```python
from build123d import *

# Parameters (mm, degrees)
F0_W     = 83
F0_H     = 60
F1_DEPTH = 25
F2_R     = 5
F3_SIZE  = 10
F5_D     = 4.2
F6_W     = 9.244158864
F6_H     = 29.9456948414
F7_DEPTH = 30
F8_W     = 29.5899156481
F8_H     = 11.4948265254
F9_DEPTH = 15


with BuildPart() as f1:
    # F0 (on Top) → F1 (new body)
    with BuildSketch(Plane.XY):
        with Locations((41.5, 30)):
            Rectangle(F0_W, F0_H)
    extrude(amount=F1_DEPTH)

    # F2
    f2_edges = [f1.edges().sort_by_distance(p)[0] for p in [
        (41.5, 0, 25),
    ]]
    fillet(f2_edges, radius=F2_R)

    # F3
    f3_edges = [f1.edges().sort_by_distance(p)[0] for p in [
        (41.5, 60, 25),
    ]]
    chamfer(f3_edges, length=F3_SIZE)

    # F5 (through all)
    with Locations(Plane.XY.offset(25)):
        with Locations((41.1825105548, 21.0945475847)):
            Hole(F5_D / 2)

    # F6 (on face) → F7 (cut)
    with BuildSketch(Plane.XY.offset(25)):
        with Locations((64.5809471607, 27.1079088561)):
            Rectangle(F6_W, F6_H)
    extrude(amount=-F7_DEPTH, mode=Mode.SUBTRACT)

    # F8 (on face) → F9 (cut)
    with BuildSketch(Plane.XY.offset(25)):
        with Locations((14.7949578241, 18.5050182045)):
            Rectangle(F8_W, F8_H)
    extrude(amount=-F9_DEPTH, mode=Mode.SUBTRACT)


solid = f1.part
```
Geometry check sheet. Reference: the model listing, model coordinates, mm. A direction names the side the tool comes from. Give positions to 0.01 mm unless a question says otherwise; leave off trailing zeros. Order: outer loops, then holes, each group sorted by start corner. A loop starts at its lowest first (then second) coordinate and runs counter-clockwise, first axis right, second up.
1. Section check D-D, the plane x = 25.5. Enter the section's corners in (y, z), and give its area (3 significant figures).
2. Section check B-B, the plane x = 68. Enter the section's corners in (y, z).
3. Section check C-C, the plane z = 18.5. Enter the section's corners in (x, y).
4. Access from +Z, -Z, +X, -X, +Y, -Y to the whole of each face (thin tool, end or side, straight path). Record for faces 4 (the face through (15, 12.758, 18)), 5 (the face through (83, 30, 12)), 6 (the face through (65, 42.081, 13)).
5. Thickness scan on L1, parallel to X at y = 23.5, z = 22.75; L2, parallel to X at y = 31, z = 4.75; L3, parallel to Y at x = 28.5, z = 11.5. Record the ranges inside material, lowest first.
6. Section check A-A, the plane y = 31. Enter the section's corners in (x, z).
7. Gauge pin test, flat ends, axial feed: pin 1 Ø4 at (x, z) = (49, 19.5) entering from +Y; pin 2 Ø3.5 at (x, y) = (15.5, 16) entering from +Z; pin 3 Ø2 at (x, y) = (56, 51.5) entering from +Z. Record the tip position at first contact, or that the pin passes through.
8. Release check for a two-part mould opening along Y. For faces 1 (the face through (42, 1, 23)), 2 (the face through (41, 60, 7)), 3 (the face through (15, 19, 10)) record: pulls with the +Y half, pulls with the -Y half, needs draft (parallel to the pull), parting line crosses it, or undercut.
Values follow:
1. outline: (0, 0) - (60, 0) - (60, 15) - (50, 25) - (24.25, 25) - (24.25, 10) - (12.76, 10) - (12.76, 25) - (5, 25) arc R5 ccw to (0, 20) - close
1. area: 1,270 mm2
2. outline: (0, 0) - (12.14, 0) - (12.14, 25) - (5, 25) arc R5 ccw to (0, 20) - close; (42.08, 0) - (60, 0) - (60, 15) - (50, 25) - (42.08, 25) - close
3. outline: (0, 0) - (83, 0) - (83, 56.5) - (0, 56.5) - (0, 24.25) - (29.59, 24.25) - (29.59, 12.76) - (0, 12.76) - close; hole circle Ø4.2 at (41.18, 21.09); hole (59.96, 12.14) - (69.2, 12.14) - (69.2, 42.08) - (59.96, 42.08) - close
4. face 4: +Z, -X
4. face 5: +Z, -Z, +X, +Y, -Y
4. face 6: +Z, -Z
5. L1: x = 29.59 to 59.96, 69.2 to 83
5. L2: x = 0 to 59.96, 69.2 to 83
5. L3: y = 0 to 12.76, 24.25 to 60
6. outline: (0, 0) - (59.96, 0) - (59.96, 25) - (0, 25) - close; (69.2, 0) - (83, 0) - (83, 25) - (69.2, 25) - close
7. pin 1: stops at y = 57.5
7. pin 2: stops at z = 10
7. pin 3: stops at z = 24.5
8. face 1: pulls with the -Y half
8. face 2: pulls with the +Y half
8. face 3: undercut
